Part model, mm, in its own coordinate system. Face numbers are marked on the shaded views. A direction names the side the tool comes from. Round coordinates to 2 decimals unless told otherwise and drop trailing zeros. Write each loop counter-clockwise with the first axis right and the second up, starting at its lowest first coordinate (ties: lowest second). Pieces come first, ordered by that corner, then holes.
1) Saw through at D-D on x = -6. Write the cut outline in (y, z), and give its area (3 significant figures).
2) Which spindle directions (+Z, -Z, +X, -X, +Y, -Y) get a long thin tool onto all of the face, cutting with end or side? Do the marked faces 4, 5, 6, 7 and 8. Say none if no direction does.
3) Saw through at A-A on z = 18.25. Write the cut outline in (x, y).
4) Saw through at C-C on z = 9. Write the cut outline in (x, y).
5) Drill centre lines: L1, parallel to X at y = 0, z = 1.25; L2, parallel to Y at x = -3, z = 13; L3, parallel to Y at x = -0.5, z = 16.5. Where is each one in solid material? Low to high.
6) Saw through at B-B on y = 1. Write the cut outline in (x, z), and give its area (3 significant figures).
7) Pull direction Y, two halves, no side cores. Call the marked faces 1, 2 and 3: +Y half, -Y half, draft (parallel to the pull), parting line (faces both ways), or undercut.
8) Flat gauge pins, fed straight in: pin 1 (4 mm diameter, centred on x = 8, y = -0.5, fed in from +Z); pin 2 (5.5 mm diameter, centred on x = -5, y = 2, fed in from +Z); pin 3 (0.9 mm diameter, centred on y = 7, z = 17, fed in from -X); pin 4 (1.5 mm diameter, centred on x = 11, z = 17, fed in from +Y). Where does each tip first touch, or does it go through?
```python
from build123d import *

# Parameters (mm, degrees)
SKETCH1_W           = 24.5
SKETCH1_H           = 18
SKETCH1_W_2         = 14.5
SKETCH1_H_2         = 8
BOSS_EXTRUDE1_DEPTH = 15.5
FILLET1_R           = 5
SKETCH3_W           = 10
SKETCH3_H           = 3
SKETCH3_W_2         = 3
SKETCH3_H_2         = 4
BOSS_EXTRUDE2_DEPTH = 4.3


with BuildPart() as part:
    # Sketch1 → Boss-Extrude1 (new body)
    with BuildSketch(Plane.XY):
        Rectangle(SKETCH1_W, SKETCH1_H)
        Rectangle(SKETCH1_W_2, SKETCH1_H_2, mode=Mode.SUBTRACT)
    extrude(amount=BOSS_EXTRUDE1_DEPTH)

    # Fillet1
    fillet1_edges = [part.edges().sort_by_distance(p)[0] for p in [
        (-12.25, 9, 7.75),
        (12.25, 9, 7.75),
        (12.25, -9, 7.75),
        (-12.25, -9, 7.75),
    ]]
    fillet(fillet1_edges, radius=FILLET1_R)

    # Sketch3 → Boss-Extrude2 (add)
    with BuildSketch(Plane.XY.offset(15.5)):
        with Locations((0, -7.5)):
            Rectangle(SKETCH3_W, SKETCH3_H)
        with Locations((0, 7.5)):
            Rectangle(SKETCH3_W, SKETCH3_H)
        with Locations((-10.75, 0)):
            Rectangle(SKETCH3_W_2, SKETCH3_H_2)
        with Locations((10.75, 0)):
            Rectangle(SKETCH3_W_2, SKETCH3_H_2)
    extrude(amount=BOSS_EXTRUDE2_DEPTH)


solid = part.part
```
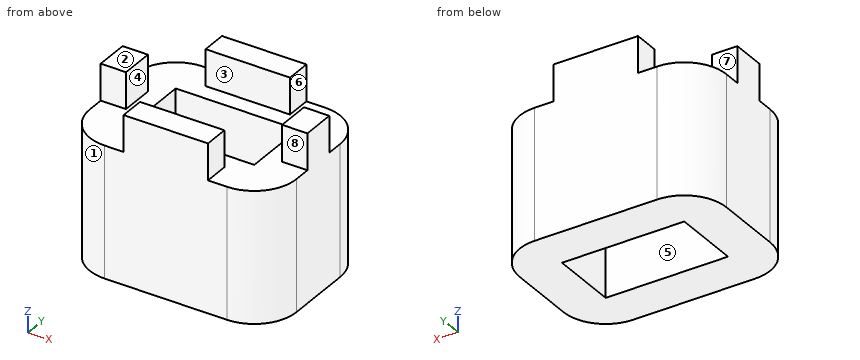
Completed:
1. outline: (-9, 0) - (-4, 0) - (-4, 15.5) - (-9, 15.5) - close; (4, 0) - (9, 0) - (9, 15.5) - (4, 15.5) - close
1. area: 155 mm2
2. face 4: +Z, +Y, -Y
2. face 5: +Z, -Z
2. face 6: +Z, +X, +Y, -Y
2. face 7: +Z, +X, -X, +Y
2. face 8: +Z, +X, -X, -Y
3. outline: (-12.25, -2) - (-9.25, -2) - (-9.25, 2) - (-12.25, 2) - close; (-5, -9) - (5, -9) - (5, -6) - (-5, -6) - close; (-5, 6) - (5, 6) - (5, 9) - (-5, 9) - close; (9.25, -2) - (12.25, -2) - (12.25, 2) - (9.25, 2) - close
4. outline: (-12.25, -4) arc R5 ccw to (-7.25, -9) - (7.25, -9) arc R5 ccw to (12.25, -4) - (12.25, 4) arc R5 ccw to (7.25, 9) - (-7.25, 9) arc R5 ccw to (-12.25, 4) - close; hole (-7.25, -4) - (7.25, -4) - (7.25, 4) - (-7.25, 4) - close
5. L1: x = -12.25 to -7.25, 7.25 to 12.25
5. L2: y = -9 to -4, 4 to 9
5. L3: y = -9 to -6, 6 to 9
6. outline: (-12.25, 0) - (-7.25, 0) - (-7.25, 15.5) - (-9.25, 15.5) - (-9.25, 19.8) - (-12.25, 19.8) - close; (7.25, 0) - (12.25, 0) - (12.25, 19.8) - (9.25, 19.8) - (9.25, 15.5) - (7.25, 15.5) - close
6. area: 181 mm2
7. face 1: -Y half
7. face 2: draft
7. face 3: undercut
8. pin 1: stops at z = 19.8
8. pin 2: stops at z = 15.5
8. pin 3: stops at x = -5
8. pin 4: stops at y = 2
